Design review of the part built by this model. Coordinates are the model's own, in mm. A direction names the side the tool comes from. Give positions to 0.01 mm unless a question says otherwise; leave off trailing zeros. Write each loop counter-clockwise with the first axis right and the second up, starting at its lowest first coordinate (ties: lowest second). Pieces come first, ordered by that corner, then holes. Notation, with made-up numbers: (58, 32.25) - (105, 32.25) arc R31 cw to (105, 64.25) - close; hole circle Ø7 at (50, 20). An arc over 180 degrees is marked (long way). Write each question's results on one line, items separated by ' | '. Start each with the question number.
Autodesk Inventor part; units mm, degrees
ref_plane "YZ Plane" through (0, 0, 0) normal (1, 0, 0) x (0, 1, 0)
ref_plane "XZ Plane" through (0, 0, 0) normal (0, 1, 0) x (-1, 0, 0)
ref_plane "XY Plane" through (0, 0, 0) normal (0, 0, 1) x (1, 0, 0)
sketch "Sketch1" plane through (0, 0, 0) normal (0, 0, 1) x (1, 0, 0)
  line L0 (-20, 0) -> (20, 0)
  line L1 (20, 0) -> (20, 27.1)
  line L2 (20, 27.1) -> (27.4, 27.1)
  line L3 (27.4, 27.1) -> (27.4, 29.6)
  line L4 (27.4, 29.6) -> (20, 29.6)
  line L5 (20, 29.6) -> (20, 37.9)
  line L6 (20, 37.9) -> (-20, 37.9)
  line L7 (-20, 37.9) -> (-20, 29.6)
  line L8 (-20, 29.6) -> (-27.4, 29.6)
  line L9 (-27.4, 29.6) -> (-27.4, 27.1)
  line L10 (-27.4, 27.1) -> (-20, 27.1)
  line L11 (-20, 27.1) -> (-20, 0)
  point P0 (0, 0)
  point P1 (0, 0)
  dimension "d0" = 40
  dimension "d1" = 27.1
  dimension "d2" = 7.4
  dimension "d3" = 2.5
  dimension "d4" = 8.3
  dimension "d5" = 7.4
extrude "Extrusion1" add sketch "Sketch1" along normal mid plane 20
sketch "Sketch4" plane through (0, 0, 0) normal (0, 0, 1) x (1, 0, 0)
  line L0 (20, 37.9) -> (-20, 37.9)
  line L1 (12.5, 37.9) -> (12.5, 42.3)
  line L2 (12.5, 42.3) -> (20.1, 42.3)
  line L3 (20.1, 42.3) -> (20.1, 45.3)
  line L4 (20.1, 45.3) -> (12.5, 45.3)
  line L5 (12.5, 45.3) -> (12.5, 45.7)
  line L6 (12.5, 45.7) -> (9.7, 45.7)
  line L7 (12.5, 37.9) -> (9.7, 37.9)
  line L8 (9.7, 45.7) -> (9.7, 37.9)
  point P0 (0, 0)
  point P1 (0, 37.9)
  dimension "d10" = 9.7
  dimension "d11" = 0.4
  dimension "d12" = 10.4
  dimension "d13" = 2.8
  dimension "d14" = 4.4
  dimension "d15" = 3
revolve "Revolution1" add sketch "Sketch4" angle 360 about axis through (9.7, 45.7, 0) along (0, -1, 0)
sketch "Sketch5" plane through (-27.4, 29.6, 10) normal (0, 1, 0) x (1, 0, 0)
  circle A0 centre (2.65, 15) radius 2
  line L0 (0, 20) -> (0, 0)
  line L1 (7.4, 0) -> (0, 0)
  line L2 (7.4, 20) -> (7.4, 0)
  line L3 (0, 20) -> (7.4, 20)
  line L4 (47.4, 20) -> (47.4, 0)
  line L5 (54.8, 0) -> (47.4, 0)
  line L6 (54.8, 20) -> (54.8, 0)
  line L7 (47.4, 20) -> (54.8, 20)
  line L8 (7.4, 20) -> (47.4, 20)
  line L9 (27.4, 20) -> (27.4, 0) construction
  line L10 (7.4, 0) -> (47.4, 0)
  line L11 (0, 20) -> (0, 0)
  line L12 (0, 10) -> (54.8, 10) construction
  line L13 (54.8, 20) -> (54.8, 0)
  circle A1 centre (2.65, 5) radius 2
  circle A2 centre (52.15, 15) radius 2
  circle A3 centre (52.15, 5) radius 2
  line L14 (7.4, 0) -> (7.4, 20)
  line L15 (7.4, 10.75) -> (0, 10.75)
  line L16 (0, 10.75) -> (0, 9.25)
  line L17 (0, 9.25) -> (7.4, 9.25)
  line L18 (7.4, 9.25) -> (7.4, 10.75)
  line L19 (47.4, 10.75) -> (54.8, 10.75)
  line L20 (54.8, 10.75) -> (54.8, 9.25)
  line L21 (54.8, 9.25) -> (47.4, 9.25)
  line L22 (47.4, 9.25) -> (47.4, 10.75)
  point P0 (27.4, 10)
  dimension "d17" = 4
  dimension "d18" = 10
  dimension "d19" = 49.5
  dimension "d22" = 7.4
  dimension "d23" = 1.5
extrude "Extrusion2" cut sketch "Sketch5" against normal up to next contours A0 | A1 | A2 | A3
extrude "Extrusion3" add sketch "Sketch5" along normal blind 1 contours L15 L2 L17 L0 | L19 L6 L21 L4
sketch "Sketch6" plane through (-20, 0, 10) normal (0, -1, 0) x (1, 0, 0)
  line L0 (0, 0) -> (0, -20) construction
  line L1 (0, -10) -> (40, -10) construction
  line L2 (40, -20) -> (40, 0) construction
  line L3 (40, 0) -> (0, 0) construction
  line L4 (20, 0) -> (20, -20) construction
  line L5 (0, -20) -> (40, -20) construction
  line L6 (40, 0) -> (0, 0) construction
  line L7 (0, 0) -> (0, -20) construction
  line L8 (0, -20) -> (40, -20) construction
  line L9 (40, -20) -> (40, 0) construction
  circle A0 centre (29.7, -10) radius 2.8
  circle A1 centre (-4.75, -5) radius 2
  circle A2 centre (-4.75, -15) radius 2
  circle A3 centre (44.75, -15) radius 2
  circle A4 centre (44.75, -5) radius 2
  point P0 (20, -10)
  point P1 (29.7, -10)
properties part number "FS5106B_servo"
Q1. Add section C-C on x = 24.75. State the section outline as (y, z) points.
Q2. Add section B-B on z = 6. State the section outline as (x, y) points.
Q3. Add section A-A on x = 15. State the section outline as (y, z) points, plus the area to 3 significant figures.
Q4. The part is to be moulded in two halves that separate along Y. For faces 1 (the face through (20, 13, 0)), 2 (the face through (10, 45.7, 0)), 3 (the face through (12, 42.3, -2)), say which applies: +Y half, -Y half, draft (parallel to the pull), parting line (faces both ways), or undercut.
Q5. For line 1 along X through (y, z) = (28.9, 5); line 2 along Z through (x, y) = (24.75, 28.6); line 3 along Y through (x, z) = (14, 8.25), list the stretches that pass through material, from the lowest coordinate up. Write a range as [from, to].
Q6. Insertion check: P1, Ø3, axis at x = -24.75, z = 5, coming from the -Y side; P2, Ø2, axis at x = -19, y = 16, coming from the +Z side; P3, Ø4, axis at y = 32.5, z = 2.5, coming from the -X side; P4, Ø5, axis at x = -24.75, z = -5, coming from the -Y side. Each pin has a flat end and moves straight along its axis. Give the tip position at first contact, or say it passes through.
Q7. Machinability: for faces 4 (the face through (-22.8, 29.6, -6.5)), 5 (the face through (6.9, 45.5, -0.1)), 6 (the face through (0, 19, 10)), 7 (the face through (-24, 30.6, 0)), which of the approach directions +Z, -Z, +X, -X, +Y, -Y give a long, thin tool a straight path to every point of the face, cutting with its end or side? Answer none if there is none.
Q8. Add section D-D on z = 0. State the section outline as (x, y) points.
Result:
1) outline: (27.1, -10) - (29.6, -10) - (29.6, -7) - (27.1, -7) - close; (27.1, -3) - (29.6, -3) - (29.6, -0.75) - (30.6, -0.75) - (30.6, 0.75) - (29.6, 0.75) - (29.6, 3) - (27.1, 3) - close; (27.1, 7) - (29.6, 7) - (29.6, 10) - (27.1, 10) - close
2) outline: (-27.4, 27.1) - (-26.48, 27.1) - (-26.48, 29.6) - (-27.4, 29.6) - close; (-23.02, 27.1) - (-20, 27.1) - (-20, 0) - (20, 0) - (20, 27.1) - (23.02, 27.1) - (23.02, 29.6) - (20, 29.6) - (20, 37.9) - (-20, 37.9) - (-20, 29.6) - (-23.02, 29.6) - close; (1.21, 42.3) - (18.19, 42.3) - (18.19, 45.3) - (1.21, 45.3) - close; (26.48, 27.1) - (27.4, 27.1) - (27.4, 29.6) - (26.48, 29.6) - close
3) outline: (0, -10) - (37.9, -10) - (37.9, 10) - (0, 10) - close; (42.3, -8.95) - (45.3, -8.95) - (45.3, 8.95) - (42.3, 8.95) - close | area: 812 mm²
4) face 1: draft | face 2: +Y half | face 3: undercut
5) line 1: x = [-27.4, -26.75], [-22.75, 22.75], [26.75, 27.4] | line 2: z = [-10, -7], [-3, 3], [7, 10] | line 3: y = [0, 37.9], [42.3, 45.3]
6) P1: passes through | P2: stops at z = 10 | P3: stops at x = -20 | P4: stops at y = 27.1
7) face 4: -Z, -X, +Y | face 5: +Y | face 6: +Z, +X, -X, -Y | face 7: +Z, -Z, -X, +Y
8) outline: (-27.4, 27.1) - (-20, 27.1) - (-20, 0) - (20, 0) - (20, 27.1) - (27.4, 27.1) - (27.4, 30.6) - (20, 30.6) - (20, 37.9) - (12.5, 37.9) - (12.5, 42.3) - (20.1, 42.3) - (20.1, 45.3) - (12.5, 45.3) - (12.5, 45.7) - (6.9, 45.7) - (6.9, 45.3) - (-0.7, 45.3) - (-0.7, 42.3) - (6.9, 42.3) - (6.9, 37.9) - (-20, 37.9) - (-20, 30.6) - (-27.4, 30.6) - close
